from build123d import *

# Parameters (mm, degrees)
EXTRUDE_1_DEPTH        = 280
HOLE_WIZARD_M6_3_D     = 5
HOLE_WIZARD_M6_3_DEPTH = 17
HOLE_WIZARD_M6_3_TIP   = 1.502151548
HOLE_WIZARD_M6_4_D     = 5
HOLE_WIZARD_M6_4_DEPTH = 17
HOLE_WIZARD_M6_4_TIP   = 1.502151548


with BuildPart() as part:
    # 草图1 → 凸台-拉伸1 (new body)
    with BuildSketch(Plane(origin=(0, 0, 0), x_dir=(1, 0, 0), z_dir=(0, 1, 0))):
        Polygon((-119.239761807, 232.240117312), (-89.239761807, 232.240117312), (-89.239761807, 228.470843435), (-115.239761807, 228.470843435), (-115.239761807, 201.561077594), (-119.239761807, 201.561077594), (-119.239761807, 228.23121253), align=None)
    extrude(amount=EXTRUDE_1_DEPTH)

    # M6 螺纹孔3
    with Locations(Plane.ZY.offset(119.239761807)):
        with Locations((-213.240117312, 10), (-213.240117312, 270)):
            Hole(HOLE_WIZARD_M6_3_D / 2, depth=HOLE_WIZARD_M6_3_DEPTH)
            with Locations((0, 0, -(HOLE_WIZARD_M6_3_DEPTH + HOLE_WIZARD_M6_3_TIP / 2))):  # 118° drill point
                Cone(0, HOLE_WIZARD_M6_3_D / 2, HOLE_WIZARD_M6_3_TIP, mode=Mode.SUBTRACT)

    # M6 螺纹孔4
    with Locations(Plane(origin=(0, 0, -232.240117312), x_dir=(-1, 0, 0), z_dir=(0, 0, -1))):
        with Locations((100.239761807, 10), (100.239761807, 270)):
            Hole(HOLE_WIZARD_M6_4_D / 2, depth=HOLE_WIZARD_M6_4_DEPTH)
            with Locations((0, 0, -(HOLE_WIZARD_M6_4_DEPTH + HOLE_WIZARD_M6_4_TIP / 2))):  # 118° drill point
                Cone(0, HOLE_WIZARD_M6_4_D / 2, HOLE_WIZARD_M6_4_TIP, mode=Mode.SUBTRACT)


solid = part.part
Part model, mm, in its own coordinate system. A direction names the side the tool comes from. Give positions to 0.01 mm unless a question says otherwise; leave off trailing zeros. Order: outer loops, then holes, each group sorted by start corner. A loop starts at its lowest first (then second) coordinate and runs counter-clockwise, first axis right, second up. Notation, with made-up numbers: (54, -28.5) - (77, -28.5) arc R16 cw to (77, -12.5) - close; hole circle Ø5 at (19, 61). An arc over 180 degrees is marked (long way). One line per question, with ' | ' between items.
1. Band-saw the part on B-B on z = -207. List the corners of the cut face in (x, y), then the cut area to 3 significant figures.
Filled in:
outline: (-119.24, 0) - (-115.24, 0) - (-115.24, 280) - (-119.24, 280) - close | area: 1,120 mm²
2. Drill centre lines: probe 1 along X at (y, z) = (185, -203.5); probe 2 along Z at (x, y) = (-110, 26); probe 3 along X at (y, z) = (270, -231). Where is each one in solid material? Low to high.
Filled in:
probe 1: -119.24 to -115.24 | probe 2: -232.24 to -228.47 | probe 3: -119.24 to -102.74, -97.74 to -89.24
3. Band-saw the part on C-C on y = 40. List the corners of the cut face in (x, z), then the cut area to 3 significant figures.
Filled in:
outline: (-119.24, -232.24) - (-89.24, -232.24) - (-89.24, -228.47) - (-115.24, -228.47) - (-115.24, -201.56) - (-119.24, -201.56) - close | area: 221 mm²
4. Which spindle directions (+Z, -Z, +X, -X, +Y, -Y) get a long thin tool onto all of the face, cutting with end or side? Do faces 1 (the face through (-117.21, 271.69, -211.4)), 2 (the face through (-102, 138, -228.471)). Say none if no direction does.
Filled in:
face 1: +X, -X | face 2: +Z, +X, +Y, -Y
5. Drop a flat-ended pin along its axis: P1, Ø6, axis at x = -107.5, y = 132.5, coming from the +Z side. Give the stop position or say it passes through.
Filled in:
P1: z = -228.47
6. Band-saw the part on A-A on y = 270. List the corners of the cut face in (x, z).
Filled in:
outline: (-119.24, -232.24) - (-102.74, -232.24) - (-102.74, -228.47) - (-115.24, -228.47) - (-115.24, -215.74) - (-119.24, -215.74) - close; (-119.24, -210.74) - (-115.24, -210.74) - (-115.24, -201.56) - (-119.24, -201.56) - close; (-97.74, -232.24) - (-89.24, -232.24) - (-89.24, -228.47) - (-97.74, -228.47) - close
7. Band-saw the part on D-D on x = -107. List the corners of the cut face in (y, z), then the cut area to 3 significant figures.
Filled in:
outline: (0, -232.24) - (280, -232.24) - (280, -228.47) - (0, -228.47) - close | area: 1,060 mm²
8. Pull direction X, two halves, no side cores. Call faces 3 (the face through (-100.57, 272.48, -230.33)), 4 (the face through (-116, 280, -223)), 5 (the face through (-115.24, 138, -215)): +X half, -X half, draft (parallel to the pull), parting line (faces both ways), or undercut.
Filled in:
face 3: undercut | face 4: draft | face 5: +X half
